Autodesk Inventor part; units mm, degrees
ref_plane "YZ Plane" through (0, 0, 0) normal (1, 0, 0) x (0, 1, 0)
ref_plane "XZ Plane" through (0, 0, 0) normal (0, 1, 0) x (-1, 0, 0)
ref_plane "XY Plane" through (0, 0, 0) normal (0, 0, 1) x (1, 0, 0)
sketch "Sketch1" plane through (0, 0, 0) normal (0, 1, 0) x (-1, 0, 0)
  line L0 (-50, -27.5) -> (-50, -52.5)
  line L1 (-50, -52.5) -> (0, -52.5)
  line L2 (0, 52.5) -> (-50, 52.5)
  line L3 (-50, 52.5) -> (-50, 27.5)
  line L4 (-50, 27.5) -> (-5.8866, 27.5)
  line L5 (-5.8866, -27.5) -> (-50, -27.5)
  line L6 (-5.8866, 27.5) -> (-5.8866, -27.5)
  line L7 (0, -52.5) -> (0, 52.5)
  point P0 (0, 0)
revolve "Revolution1" add sketch "Sketch1" angle 360 about axis through (0, 0, -52.5) along (0, 0, 1)
fillet "Fillet1" radius 10 4 edges at (-50, 0, 27.5) (-50, 0, -27.5) (-50, 0, -52.5) (-50, 0, 52.5)
properties part number "WHEEL"
Here's how the part is built. I have some questions about the finished solid (model axes, mm). A direction names the side the tool comes from. Round coordinates to 2 decimals unless told otherwise and drop trailing zeros. Loops run counter-clockwise (first coordinate to the right, second up) from the corner with the lowest first, then second, coordinate; pieces in that order, holes last.
1. If I drill on line 1 along Z through (x, y) = (-29.5, -5); line 2 along Z through (x, y) = (21.5, -39.5); line 3 along X through (y, z) = (1.5, 36), over which ranges is the centre line in solid material (lowest first)?
Answer list:
line 1: z = -52.5 to -27.5, 27.5 to 52.5
line 2: z = -51.18 to -28.82, 28.82 to 51.18
line 3: x = -49.86 to 49.86
2. If we section it at A-A on y = 0: Write out the boundary of the cut face in (x, z), plus the area to 3 significant figures.
Answer list:
outline: (-50, -42.5) arc R10 ccw to (-40, -52.5) - (40, -52.5) arc R10 ccw to (50, -42.5) - (50, -37.5) arc R10 ccw to (40, -27.5) - (5.89, -27.5) - (5.89, 27.5) - (40, 27.5) arc R10 ccw to (50, 37.5) - (50, 42.5) arc R10 ccw to (40, 52.5) - (-40, 52.5) arc R10 ccw to (-50, 42.5) - (-50, 37.5) arc R10 ccw to (-40, 27.5) - (-5.89, 27.5) - (-5.89, -27.5) - (-40, -27.5) arc R10 ccw to (-50, -37.5) - close
area: 5,480 mm2
3. If we section it at D-D on z = -32.5: Write out the boundary of the cut face in (x, y).
Answer list:
outline: circle Ø97.32 at (0, 0)
4. We'd pull the mould along Z, two halves only. Please class faces 1 (the face through (-1, 1, -52.5)), 2 (the face through (47.69, -15.02, 39.97)), 3 (the face through (8, 1, 27.5)): +Z half, -Z half, draft (parallel to the pull), parting line (faces both ways), or undercut.
Answer list:
face 1: -Z half
face 2: draft
face 3: undercut
5. For P1, Ø8, axis at x = 1, z = -19.5, coming from the +Y side; P2, Ø3, axis at y = 0.5, z = -15.5, coming from the +X side, each with a flat end and sliding along its axis, tell me the tip position at first contact or that it passes through.
Answer list:
P1: stops at y = 5.89
P2: stops at x = 5.89
6. Which directions (+Z, -Z, +X, -X, +Y, -Y) give clear straight access to the entire face, cutting with the end or side of a thin tool? Please do faces 4 (the face through (5.615, -1.768, -0.385)), 5 (the face through (-1, 1, 52.5)).
Answer list:
face 4: none
face 5: +Z, +X, -X, +Y, -Y
7. If we section it at C-C on z = 5.5: Write out the boundary of the cut face in (x, y), plus the area to 3 significant figures.
Answer list:
outline: circle Ø11.77 at (0, 0)
area: 109 mm2
